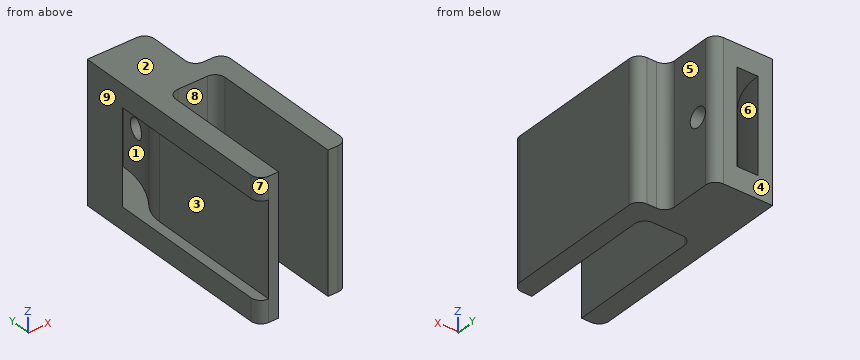
from build123d import *

# Parameters (mm, degrees)
BOSS_EXTRUDE3_DEPTH = 14
SKETCH5_W           = 9.5
SKETCH5_H           = 3
SKETCH9_R           = 0.975
CUT_EXTRUDE1_DEPTH  = 4.5
CUT_EXTRUDE3_DEPTH  = 1
FILLET2_R           = 4


with BuildPart() as part:
    # Sketch4 → Boss-Extrude3 (new body)
    with BuildSketch(Plane.XY):
        with BuildLine():
            Line((7, -16), (8, -16))
            ThreePointArc((8, -16), (8.707106781, -15.707106781), (9, -15))
            Line((9, -15), (9, -1))
            ThreePointArc((9, -1), (8.707106781, -0.292893219), (8, 0))
            Line((8, 0), (7, 0))
            ThreePointArc((7, 0), (6.292893219, 0.292893219), (6, 1))
            Line((6, 1), (6, 5))
            ThreePointArc((6, 5), (5.707106781, 5.707106781), (5, 6))
            Line((5, 6), (0, 6))
            Line((0, 6), (0, 0))
            Line((0, 0), (0, -15))
            ThreePointArc((0, -15), (0.292893219, -15.707106781), (1, -16))
            Line((1, -16), (2, -16))
            Line((2, -16), (2, -2.806818182))
            ThreePointArc((2, -2.806818182), (2.292893219, -2.099711401), (3, -1.806818182))
            Line((3, -1.806818182), (6, -1.806818182))
            ThreePointArc((6, -1.806818182), (6.707106781, -2.099711401), (7, -2.806818182))
            Line((7, -2.806818182), (7, -16))
        make_face()
    extrude(amount=BOSS_EXTRUDE3_DEPTH)

    # Cut-Sweep2: sweep along a path in Sketch8
    with BuildLine(Plane.XY.offset(14)) as cut_sweep2_path:
        CenterArc((-6, 6), 11, 0, 360)
    # Sketch5 → Cut-Sweep2 (sweep, cut)
    with BuildSketch(Plane.ZY):
        with Locations((7, 0)):
            Rectangle(SKETCH5_W, SKETCH5_H)
    sweep(path=cut_sweep2_path.line, mode=Mode.SUBTRACT)

    # Sketch9 → Cut-Extrude1 (cut)
    with BuildSketch(Plane(origin=(6, 0, 0), x_dir=(0, 0, -1), z_dir=(1, 0, 0))):
        with Locations((-7, 4)):
            Circle(SKETCH9_R)
    extrude(amount=-CUT_EXTRUDE1_DEPTH, mode=Mode.SUBTRACT)

    # Sketch11 → Cut-Extrude3 (cut)
    with BuildSketch(Plane.ZY):
        Polygon((2.25, -1.5), (2.25, 0), (11.75, 0), (11.75, -1.5), (11.75, -16), (2.25, -16), align=None)
    extrude(amount=-CUT_EXTRUDE3_DEPTH, mode=Mode.SUBTRACT)

    # Fillet2
    fillet2_edges = [part.edges().sort_by_distance(p)[0] for p in [
        (1, -0.576473219, 7),
    ]]
    fillet(fillet2_edges, radius=FILLET2_R)


solid = part.part
Design review of the part built by this model. Coordinates are the model's own, in mm. Face numbers are marked on the shaded views. A direction names the side the tool comes from. Coordinates: 2 decimals unless noted, no trailing zeros. Loops run counter-clockwise (first coordinate to the right, second up) from the corner with the lowest first, then second, coordinate; pieces in that order, holes last. Notation, with made-up numbers: M -38.5,77.25 L 8.5,77.25 A13 cw 8.5,98.25 Z; hole C 69.5,-40 d11. An arc over 180 degrees is marked long. Answer as CSV lines item,"result".
Item 1: The part is to be moulded in two halves that separate along Z. For the marked faces 1, 2, 3 and 4, say which applies: pulls with the +Z half, pulls with the -Z half, needs draft (parallel to the pull), parting line crosses it, or undercut.
Answer list:
face 1,"undercut"
face 2,"pulls with the +Z half"
face 3,"undercut"
face 4,"needs draft"
Item 2: Add section D-D on z = 7.75. State the section outline as (x, y) points, plus the area to 3 significant figures.
Answer list:
outline,"M 0,1.5 A7.5 ccw 1.5,6 L 0,6 Z; M 1,-16 L 2,-16 L 2,-2.81 A1 cw 3,-1.81 L 6,-1.81 A1 cw 7,-2.81 L 7,-16 L 8,-16 A1 ccw 9,-15 L 9,-1 A1 ccw 8,0 L 7,0 A1 cw 6,1 L 6,3.38 L 3.24,3.38 A9.6 cw 1.77,0.35 A4 ccw 1,-2.01 Z; M 3.51,4.62 L 6,4.62 L 6,5 A1 ccw 5,6 L 3.6,6 A9.6 cw Z"
area,"76.4 mm²"
Item 3: For probe 1 along Z at (x, y) = (4.2, 4) (3 decimals); probe 2 along Y at (x, z) = (4.25, 7) (3 decimals); probe 3 along X at (y, z) = (-11.75, 10.25), list the stretches that pass through material, from the lowest coordinate up.
Answer list:
probe 1,"0 to 6.025, 7.975 to 14"
probe 2,"-1.807 to 3.025, 4.975 to 6"
probe 3,"1 to 2, 7 to 9"
Item 4: Add section B-B on y = -3.5. State the section outline as (x, z) points.
Answer list:
outline,"M 0,0 L 2,0 L 2,14 L 0,14 L 0,11.75 L 1,11.75 L 1,2.25 L 0,2.25 Z; M 7,0 L 9,0 L 9,14 L 7,14 Z"
Item 5: Add section C-C on x = 4.25. State the section outline as (y, z) points (3 decimals), plus the area to 3 significant figures.
Answer list:
outline,"M -1.807,0 L 6,0 L 6,14 L -1.807,14 Z; hole C 4,7 d1.95"
area,"106 mm²"
Item 6: For P1, Ø4.5, axis at y = 3, z = 10, coming from the +X side; P2, Ø2.5, axis at x = 5, z = 9.5, coming from the -Y side, all flat-tipped, find the tip position at first contact; note any pin that passes through.
Answer list:
P1,"x = 6.03"
P2,"y = -1.84"
Item 7: Add section A-A on z = 2.75. State the section outline as (x, y) points, plus the area to 3 significant figures.
Answer list:
outline,"M 0,1.5 A7.5 ccw 1.5,6 L 0,6 Z; M 1,-16 L 2,-16 L 2,-2.81 A1 cw 3,-1.81 L 6,-1.81 A1 cw 7,-2.81 L 7,-16 L 8,-16 A1 ccw 9,-15 L 9,-1 A1 ccw 8,0 L 7,0 A1 cw 6,1 L 6,5 A1 ccw 5,6 L 3.6,6 A9.6 cw 1.77,0.35 A4 ccw 1,-2.01 Z"
area,"79.7 mm²"
Item 8: Machinability: for the marked faces 5, 6, 7, 8 and 9, which of the approach directions +Z, -Z, +X, -X, +Y, -Y give a long, thin tool a straight path to every point of the face, cutting with its end or side? Answer none if there is none.
Answer list:
face 5,"+Z, -Z, +X, +Y"
face 6,"none"
face 7,"+Z, -Z, -X, -Y"
face 8,"+Z, -Z, -Y"
face 9,"+Z, -Z, -X, +Y, -Y"
